from build123d import *

# Parameters (mm, degrees)
SKETCH1_W           = 53.594
SKETCH1_H           = 53.594
SKETCH1_R           = 16.51
SKETCH1_R_2         = 1.7
SKETCH1_R_3         = 1.926649595
BOSS_EXTRUDE1_DEPTH = 4.7625


with BuildPart() as part:
    # Sketch1 → Boss-Extrude1 (new body)
    with BuildSketch(Plane(origin=(0, 0, 0), x_dir=(1, 0, 0), z_dir=(0, 1, 0))):
        Rectangle(SKETCH1_W, SKETCH1_H)
        Circle(SKETCH1_R, mode=Mode.SUBTRACT)
        with Locations((-15.5, 15.5)):
            Circle(SKETCH1_R_2, mode=Mode.SUBTRACT)
        with Locations((15.5, 15.5)):
            Circle(SKETCH1_R_2, mode=Mode.SUBTRACT)
        with Locations((15.5, -15.5)):
            Circle(SKETCH1_R_2, mode=Mode.SUBTRACT)
        with Locations((-15.5, -15.5)):
            Circle(SKETCH1_R_2, mode=Mode.SUBTRACT)
        with Locations((0, 23.622)):
            Circle(SKETCH1_R_3, mode=Mode.SUBTRACT)
        with Locations((23.622, 0)):
            Circle(SKETCH1_R_3, mode=Mode.SUBTRACT)
        with Locations((0, -23.622)):
            Circle(SKETCH1_R_3, mode=Mode.SUBTRACT)
        with Locations((-23.622, 0)):
            Circle(SKETCH1_R_3, mode=Mode.SUBTRACT)
    extrude(amount=BOSS_EXTRUDE1_DEPTH)


solid = part.part
Geometry check sheet. Reference: the model listing, model coordinates, mm. Round coordinates to 2 decimals unless told otherwise and drop trailing zeros. Order: outer loops, then holes, each group sorted by start corner. A loop starts at its lowest first (then second) coordinate and runs counter-clockwise, first axis right, second up. Notation, with made-up numbers: M -30,-21.5 L 28,-21.5 A29 ccw 28,10.5 Z; hole C -34.5,60.25 d4. An arc over 180 degrees is marked long. Answer in a Markdown table with one row per item.
(1) Sectioned sample at D-D, the plane y = 3.7. State how many separate pieces and enclosed holes the cut face has, and give its area (3 significant figures).
Responses:
| item | result |
|---|---|
| separate pieces | 1 |
| enclosed holes | 9 |
| area | 1,930 mm² |
(2) Go/stop test with a flat-tipped pin: P1, Ø4.5, axis at x = -15.5, z = 15.5, coming from the +Y side. Record where the tip stops, or that it passes through.
Responses:
| item | result |
|---|---|
| P1 | stops at y = 4.76 |
(3) Sectioned sample at C-C, the plane x = -15. Record the cut outline in (y, z).
Responses:
| item | result |
|---|---|
| outline | M 0,-26.8 L 4.76,-26.8 L 4.76,-17.12 L 0,-17.12 Z; M 0,-13.88 L 4.76,-13.88 L 4.76,-6.9 L 0,-6.9 Z; M 0,6.9 L 4.76,6.9 L 4.76,13.88 L 0,13.88 Z; M 0,17.12 L 4.76,17.12 L 4.76,26.8 L 0,26.8 Z |
(4) Draft check along Z on faces 1 (the face through (0, 2, 26.797)), 2 (the face through (15.748, 2.348, -4.959)), 3 (the face through (-12, 4.762, -12)). Enter one of: released by +Z, released by -Z, zero draft, split by the parting line, or undercut.
Responses:
| item | result |
|---|---|
| face 1 | released by +Z |
| face 2 | undercut |
| face 3 | zero draft |
(5) Sectioned sample at B-B, the plane x = 4. Record the cut outline in (y, z).
Responses:
| item | result |
|---|---|
| outline | M 0,-26.8 L 4.76,-26.8 L 4.76,-16.02 L 0,-16.02 Z; M 0,16.02 L 4.76,16.02 L 4.76,26.8 L 0,26.8 Z |
(6) Scan lines: probe 1 along X at (y, z) = (3.3, 0); probe 2 along Z at (x, y) = (12, 1.3); probe 3 along Z at (x, y) = (-14, 3.25). Record each from-to range of solid material in increasing order. Write a range as from..to.
Responses:
| item | result |
|---|---|
| probe 1 | x = -26.8..-25.55, -21.7..-16.51, 16.51..21.7, 25.55..26.8 |
| probe 2 | z = -26.8..-11.34, 11.34..26.8 |
| probe 3 | z = -26.8..-16.3, -14.7..-8.75, 8.75..14.7, 16.3..26.8 |
(7) Sectioned sample at A-A, the plane z = 0. Record the cut outline in (x, y).
Responses:
| item | result |
|---|---|
| outline | M -26.8,0 L -25.55,0 L -25.55,4.76 L -26.8,4.76 Z; M -21.7,0 L -16.51,0 L -16.51,4.76 L -21.7,4.76 Z; M 16.51,0 L 21.7,0 L 21.7,4.76 L 16.51,4.76 Z; M 25.55,0 L 26.8,0 L 26.8,4.76 L 25.55,4.76 Z |
